Geometry: final body of the model. Coordinates: model frame, mm. A direction names the side the tool comes from. Coordinates: 2 decimals unless noted, no trailing zeros. Order: outer loops, then holes, each group sorted by start corner. A loop starts at its lowest first (then second) coordinate and runs counter-clockwise, first axis right, second up. Notation, with made-up numbers: M 9,-37 L 13,-37 A13 cw 13,-15 Z; hole C 59.25,-6 d11. An arc over 180 degrees is marked long. Write item = value, one per line.
from build123d import *

# Parameters (mm, degrees)
CYLINDER006_R          = 2
CYLINDER006_DEPTH      = 10
CYLINDER007_R          = 2
CYLINDER007_DEPTH      = 10
CYLINDER052_R          = 2
CYLINDER052_DEPTH      = 10
CYLINDER055_R          = 2
CYLINDER055_DEPTH      = 10
CYLINDER054_R          = 4
CYLINDER054_DEPTH      = 60
CYLINDER053_R          = 7.7
CYLINDER053_DEPTH      = 40
BOX019_W               = 25
BOX019_H               = 25
BOX019_DEPTH           = 5.2
CUT004_ROLL_ANGLE      = -90
CUT004_PLACEMENT_ANGLE = -90


with BuildPart() as cylinder006:
    # Cylinder006 → Cylinder006 (new body)
    with BuildSketch(Plane(origin=(21, 21, -2), x_dir=(1, 0, 0), z_dir=(0, 0, 1))):
        Circle(CYLINDER006_R)
    extrude(amount=CYLINDER006_DEPTH)


with BuildPart() as cylinder007:
    # Cylinder007 → Cylinder007 (new body)
    with BuildSketch(Plane(origin=(21, 4, -2), x_dir=(1, 0, 0), z_dir=(0, 0, 1))):
        Circle(CYLINDER007_R)
    extrude(amount=CYLINDER007_DEPTH)


with BuildPart() as cylinder052:
    # Cylinder052 → Cylinder052 (new body)
    with BuildSketch(Plane(origin=(4, 21, -2), x_dir=(1, 0, 0), z_dir=(0, 0, 1))):
        Circle(CYLINDER052_R)
    extrude(amount=CYLINDER052_DEPTH)


with BuildPart() as cylinder055:
    # Cylinder055 → Cylinder055 (new body)
    with BuildSketch(Plane(origin=(4, 4, -2), x_dir=(1, 0, 0), z_dir=(0, 0, 1))):
        Circle(CYLINDER055_R)
    extrude(amount=CYLINDER055_DEPTH)


with BuildPart() as cylinder054:
    # Cylinder054 → Cylinder054 (new body)
    with BuildSketch(Plane(origin=(12.5, 12.5, -7), x_dir=(1, 0, 0), z_dir=(0, 0, 1))):
        Circle(CYLINDER054_R)
    extrude(amount=CYLINDER054_DEPTH)


with BuildPart() as cylinder053:
    # Cylinder053 → Cylinder053 (new body)
    with BuildSketch(Plane(origin=(12.5, 12.5, 5), x_dir=(1, 0, 0), z_dir=(0, 0, 1))):
        Circle(CYLINDER053_R)
    extrude(amount=CYLINDER053_DEPTH)


with BuildPart() as cut004:
    # Box019 → Box019 (new body)
    with BuildSketch(Plane.XY):
        with Locations((12.5, 12.5)):
            Rectangle(BOX019_W, BOX019_H)
    extrude(amount=BOX019_DEPTH)

    # Fusion022: union Cylinder053
    add(cylinder053.part)

    # Cut: cut Cylinder054
    add(cylinder054.part, mode=Mode.SUBTRACT)

    # Cut001: cut Cylinder055
    add(cylinder055.part, mode=Mode.SUBTRACT)

    # Cut002: cut Cylinder052
    add(cylinder052.part, mode=Mode.SUBTRACT)

    # Cut003: cut Cylinder007
    add(cylinder007.part, mode=Mode.SUBTRACT)

    # Cut004: cut Cylinder006
    add(cylinder006.part, mode=Mode.SUBTRACT)


with BuildPart() as cut004_1:
    # Cut004 roll: moved
    add(cut004.part.rotate(Axis((0, 0, 0), (1, 0, 0)), CUT004_ROLL_ANGLE))


with BuildPart() as cut004_2:
    # Cut004 placement: moved
    add(cut004_1.part.moved(Location((79.5, 19.5, 35.5))).rotate(Axis((79.5, 19.5, 35.5), (0, 0, 1)), CUT004_PLACEMENT_ANGLE))


solid = cut004_2.part
1) Line query: L1, parallel to Z at x = 81.6, y = 15.5; L2, parallel to Z at x = 117.5, y = 7.5; L3, parallel to X at y = 14, z = 33. Output: solid intervals per line, ascending.
Numbers:
L1 = 10.5 to 12.5, 16.5 to 29.5, 33.5 to 35.5
L2 = 15.32 to 19.03, 26.97 to 30.68
L3 = 79.5 to 84.7
2) Section D-D, the plane y = 15.5. Return loops of the section in (x, z), and give its area (3 significant figures).
Numbers:
outline = M 79.5,10.5 L 84.7,10.5 L 84.7,12.5 L 79.5,12.5 Z; M 79.5,16.5 L 84.7,16.5 L 84.7,29.5 L 79.5,29.5 Z; M 79.5,33.5 L 84.7,33.5 L 84.7,35.5 L 79.5,35.5 Z
area = 88.4 mm²
3) Section B-B, the plane y = 7. Return loops of the section in (x, z), and give its area (3 significant figures).
Numbers:
outline = M 79.5,10.5 L 84.7,10.5 L 84.7,15.3 L 124.5,15.3 L 124.5,19 L 79.5,19 Z; M 79.5,27 L 124.5,27 L 124.5,30.7 L 84.7,30.7 L 84.7,35.5 L 79.5,35.5 Z
area = 383 mm²
4) Section A-A, the plane z = 31.5. Return loops of the section in (x, y).
Numbers:
outline = M 79.5,-5.5 L 84.7,-5.5 L 84.7,-3.5 L 79.5,-3.5 Z; M 79.5,0.5 L 84.7,0.5 L 84.7,13.5 L 79.5,13.5 Z; M 79.5,17.5 L 84.7,17.5 L 84.7,19.5 L 79.5,19.5 Z
5) Set-up query: faces 4 (the face through (104.32, 12.68, 17.8)), 5 (the face through (82.064, -1.24, 12.517)). Return all of +Z, -Z, +X, -X, +Y, -Y with unobstructed straight access to the full face (end or side cutting, diameter ignored); none if empty.
Numbers:
face_4 = +X
face_5 = +X, -X
6) Pin query (flat end, axial travel): pin 1 (1 mm diameter, centred on x = 109, y = 2, fed in from +Z); pin 2 (5 mm diameter, centred on y = 15.5, z = 31.5, fed in from +X); pin 3 (10 mm diameter, centred on x = 109.5, y = 5, fed in from +Z). Return the tip coordinate at first contact, or that it passes through.
Numbers:
pin_1 = 29.25
pin_2 = 84.7
pin_3 = 30.7
7) Mould query, pull axis Z, two halves, no side actions, for faces 1 (the face through (124.5, 4, 26)), 2 (the face through (82.064, 15.76, 12.517)), 3 (the face through (82, 7, 35.5)). Classes: pulls with the +Z half, pulls with the -Z half, needs draft (parallel to the pull), parting line crosses it, or undercut.
Numbers:
face_1 = needs draft
face_2 = undercut
face_3 = pulls with the +Z half
8) Section C-C, the plane z = 23. Return loops of the section in (x, y).
Numbers:
outline = M 79.5,-5.5 L 84.7,-5.5 L 84.7,-0.7 L 124.5,-0.7 L 124.5,3 L 79.5,3 Z; M 79.5,11 L 124.5,11 L 124.5,14.7 L 84.7,14.7 L 84.7,19.5 L 79.5,19.5 Z
